from build123d import *

# Parameters (mm, degrees)
F0_W     = 58.5
F0_H     = 37.5
F0_W_2   = 4
F0_H_2   = 15
F1_DEPTH = 45
F2_T     = -1
F4_DEPTH = 52.9
F5_R     = 3.5
F6_DEPTH = 25
F7_DEPTH = 25
F8_R     = 2.5
F8_R_2   = 1.25
F9_DEPTH = 15


# Not quite as in the source:
# - a feature names something its author has since deleted; it is built from what else it names


with BuildPart() as f1:
    # F0 (on Front) → F1 (new body)
    with BuildSketch(Plane.XZ):
        with Locations((-135.4310402274, -41.6724174619)):
            Rectangle(F0_W, F0_H)
        with Locations((-159.1810402274, -44.9224174619)):
            Rectangle(F0_W_2, F0_H_2, mode=Mode.SUBTRACT)
        with Locations((-159.1810402274, -44.9224174619)):
            Rectangle(F0_W_2, F0_H_2)
    extrude(amount=F1_DEPTH)

    # F2
    f2_openings = [f1.faces().sort_by_distance(p)[0] for p in [
        (-135.43104, -45, -41.672417),
    ]]
    offset(amount=F2_T, openings=f2_openings)

    # F3 (on face) → F4 (cut)
    with BuildSketch(Plane(origin=(0, 0, -60.4224174619), x_dir=(1, 0, 0), z_dir=(0, 0, -1))):
        Polygon((-164.6810402274, 45), (-164.6810402274, 35), (-106.1810402274, 45), align=None)
    extrude(amount=-F4_DEPTH, mode=Mode.SUBTRACT)

    # F5 (on face) → F6 (cut)
    with BuildSketch(Plane.YZ.offset(-106.1810402274)):
        with Locations((-35, -32.9224174619)):
            Circle(F5_R)
    extrude(amount=-F6_DEPTH, mode=Mode.SUBTRACT)

    # F0 (on Front) → F7 (cut)
    with BuildSketch(Plane.XZ):
        with Locations((-159.1810402274, -44.9224174619)):
            Rectangle(F0_W_2, F0_H_2)
    extrude(amount=F7_DEPTH, mode=Mode.SUBTRACT)

    # F8 (on face) → F9 (join)
    with BuildSketch(Plane.XZ.offset(1)):
        with Locations((-110.1810402274, -26.9224174619)):
            Circle(F8_R)
        with Locations((-110.1810402274, -26.9224174619)):
            Circle(F8_R_2, mode=Mode.SUBTRACT)
        with Locations((-110.1810402274, -56.4224174619)):
            Circle(F8_R)
        with Locations((-110.1810402274, -56.4224174619)):
            Circle(F8_R_2, mode=Mode.SUBTRACT)
        with Locations((-160.6810402274, -56.4224174619)):
            Circle(F8_R)
        with Locations((-160.6810402274, -56.4224174619)):
            Circle(F8_R_2, mode=Mode.SUBTRACT)
        with Locations((-160.6810402274, -26.9224174619)):
            Circle(F8_R)
        with Locations((-160.6810402274, -26.9224174619)):
            Circle(F8_R_2, mode=Mode.SUBTRACT)
    extrude(amount=F9_DEPTH)


solid = f1.part
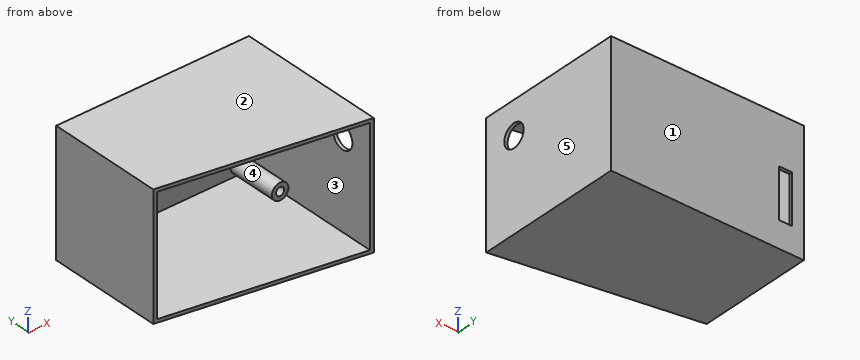
The listing builds one solid part. Answer for the finished solid, in the listing's coordinates (mm). Face numbers are marked on the shaded views. A direction names the side the tool comes from. Give positions to 0.01 mm unless a question says otherwise; leave off trailing zeros. Write each loop counter-clockwise with the first axis right and the second up, starting at its lowest first coordinate (ties: lowest second). Pieces come first, ordered by that corner, then holes. Notation, with made-up numbers: (32, 21.5) -> (59, 21.5) arc R21 cw to (59, 34.5) -> close; hole circle Ø1 at (20.25, 50.5). An arc over 180 degrees is marked (long way). Use a Markdown table: item, result.
(1) Section A-A, the plane y = -10 is taken. Give the number of separate pieces and of enclosed holes in the cut face, then the cut area to 3 significant figures.
Return value:
| item | result |
|---|---|
| separate pieces | 5 |
| enclosed holes | 5 |
| area | 247 mm2 |
(2) For the marked faces 4 and 5, determine the directions among +Z, -Z, +X, -X, +Y, -Y from which every point of the face is accessible in a straight line to the end or side of a thin tool.
Return value:
| item | result |
|---|---|
| face 4 | -Y |
| face 5 | +Z, -Z, +X, +Y, -Y |
(3) Flat-ended cylindrical pins translate along their axes: P1, Ø2, axis at x = -160.68, z = -56.42, coming from the -Y side; P2, Ø1.5, axis at x = -109.5, z = -28, coming from the -Y side; P3, Ø6, axis at y = -39, z = -31.5, coming from the -X side. Find the tip coordinate at first contact, or state that the pin passes through.
Return value:
| item | result |
|---|---|
| P1 | y = -1 |
| P2 | y = -16 |
| P3 | x = -107.18 |
(4) Section B-B, the plane z = -44.5 is taken. Determine the outline of the cut face in (x, y), then the cut area to 4 significant figures.
Return value:
| item | result |
|---|---|
| outline | (-164.68, -35) -> (-163.68, -35.17) -> (-163.68, -1) -> (-161.18, -1) -> (-161.18, 0) -> (-164.68, 0) -> close; (-157.18, -1) -> (-107.18, -1) -> (-107.18, -44.83) -> (-106.18, -45) -> (-106.18, 0) -> (-157.18, 0) -> close |
| area | 132.5 mm2 |
(5) Section D-D, the plane x = -124.5 is taken. Determine the outline of the cut face in (y, z).
Return value:
| item | result |
|---|---|
| outline | (-41.87, -60.42) -> (0, -60.42) -> (0, -22.92) -> (-41.87, -22.92) -> (-41.87, -23.92) -> (-1, -23.92) -> (-1, -59.42) -> (-41.87, -59.42) -> close |
(6) Section C-C, the plane y = -30.5 is taken. Determine the outline of the cut face in (x, z).
Return value:
| item | result |
|---|---|
| outline | (-164.68, -60.42) -> (-106.18, -60.42) -> (-106.18, -22.92) -> (-164.68, -22.92) -> close; hole (-163.68, -59.42) -> (-107.18, -59.42) -> (-107.18, -23.92) -> (-163.68, -23.92) -> close |
(7) Find the intervals of material crossed by probe 1 along X at (y, z) = (-2, -44); probe 2 along X at (y, z) = (-15.5, -57.5); probe 3 along Z at (x, y) = (-147, -36), in increasing order. Write a range as from..to.
Return value:
| item | result |
|---|---|
| probe 1 | -164.68..-163.68, -107.18..-106.18 |
| probe 2 | -164.68..-163.68, -162.94..-161.31, -160.05..-158.43, -112.44..-110.81, -109.55..-107.93, -107.18..-106.18 |
| probe 3 | -60.42..-59.42, -23.92..-22.92 |
(8) Determine the mould class of the marked faces 1, 2 and 3 for opening direction Z: released by +Z, released by -Z, zero draft, split by the parting line, or undercut.
Return value:
| item | result |
|---|---|
| face 1 | zero draft |
| face 2 | released by +Z |
| face 3 | undercut |
